Autodesk Inventor part; units mm, degrees
ref_plane "Arbeitsebene1" through (0, -13, 39.6) normal (0, 1, 0) x (-1, 0, 0)
ref_plane "YZ Plane" through (0, 0, 0) normal (1, 0, 0) x (0, 1, 0)
ref_plane "XY Plane" through (0, 0, 0) normal (0, 0, 1) x (1, 0, 0)
sketch "Skizze1" plane through (0, 0, 0) normal (0, 0, 1) x (1, 0, 0)
  circle A0 centre (0, 0) radius 15
  dimension "d0" = 30
extrude "Extrusion1" add sketch "Skizze1" along normal blind 39.6
sketch "Skizze2" plane through (0, 0, 39.6) normal (0, 0, 1) x (1, 0, 0)
  circle A0 centre (0, 0) radius 13
  dimension "d3" = 26
extrude "Extrusion2" add sketch "Skizze2" along normal blind 23
sketch "Skizze5" plane through (0, 0, 62.6) normal (0, 0, 1) x (1, 0, 0)
  circle A0 centre (0, 0) radius 9.2
  dimension "d6" = 18.4
extrude "Extrusion3" cut sketch "Skizze5" against normal through all
sketch "Skizze6" plane through (0, 0, 0) normal (0, 0, -1) x (-1, 0, 0)
  circle A0 centre (0, 0) radius 13.9
  dimension "d9" = 27.8
extrude "Extrusion4" cut sketch "Skizze6" against normal blind 20
ref_plane "Arbeitsebene1" through (0, -13, 39.6) normal (0, 1, 0) x (-1, 0, 0)
sketch "Skizze7" plane through (0, -13, 39.6) normal (0, 1, 0) x (-1, 0, 0)
  line L0 (13, 23) -> (-13, 23)
  line L1 (-9.2, 23) -> (9.2, 23) construction
  line L2 (0, 23) -> (0, 14) construction
  point P0 (0, -39.6)
  dimension "d12" = 9
hole "Bohrung1" at (0, -13, 53.6) direction (0, 1, 0) diameter 2.013 end up to surface
properties part number "tubus lense (423606-8031)"
Verification items for the finished model (mm, model axes). A direction names the side the tool comes from. Round coordinates to 2 decimals unless told otherwise and drop trailing zeros. Order: outer loops, then holes, each group sorted by start corner. A loop starts at its lowest first (then second) coordinate and runs counter-clockwise, first axis right, second up. Notation, with made-up numbers: (82.25, 80.25) -> (98.25, 80.25) arc R20 cw to (98.25, 108.25) -> close; hole circle Ø10 at (14, 31). An arc over 180 degrees is marked (long way). Put each result on its own line as item: value. Start each with the question number.
(1) Draft check along Y on faces 1 (the face through (-14.985, -0.66, 19.523)), 2 (the face through (3, 9, 62.6)), 3 (the face through (-7.3, -5.6, 41.6)). Enter one of: +Y half, -Y half, draft (parallel to the pull), parting line (faces both ways), or undercut.
(2) Section check B-B (y = 0). Enter the section's corners in (x, z).
(3) Depth check by flat-ended pin: pin 1 Ø3 at (y, z) = (2, 41.5) entering from -X; pin 2 Ø2.5 at (x, z) = (0, 53.6) entering from +Y; pin 3 Ø5 at (x, y) = (2, -4) entering from -Z; pin 4 Ø12 at (x, z) = (5, 25) entering from -Y. Enter the tip coordinate at first touch or a pass-through.
(4) Tool access check on faces 4 (the face through (-10.316, 7.91, 50.939)), 5 (the face through (10, -10, 0)), 6 (the face through (-0.3, -11.05, 52.64)), 7 (the face through (-9, -3, 20)). Record the directions out of +Z, -Z, +X, -X, +Y, -Y that give a thin tool (end or side, any length) a straight path to the whole face; none if there is none.
(5) Section check D-D (z = 50). Enter the section's corners in (x, y).
(6) Section check A-A (x = 0). Enter the section's corners in (y, z), then the cut area to 3 significant figures.
(7) Section check C-C (x = -6.25). Enter the section's corners in (y, z), then the cut area to 3 significant figures.
(8) Material ranges on line 1 along Y through (x, z) = (0.5, 56); line 2 along X through (y, z) = (5.25, 51.5); line 3 along Y through (x, z) = (4.25, 14.5), recorded low to high.
Completed:
1. face 1: parting line
1. face 2: draft
1. face 3: undercut
2. outline: (-15, 0) -> (-13.9, 0) -> (-13.9, 20) -> (-9.2, 20) -> (-9.2, 62.6) -> (-13, 62.6) -> (-13, 39.6) -> (-15, 39.6) -> close; (9.2, 20) -> (13.9, 20) -> (13.9, 0) -> (15, 0) -> (15, 39.6) -> (13, 39.6) -> (13, 62.6) -> (9.2, 62.6) -> close
3. pin 1: stops at x = -12.99
3. pin 2: stops at y = 13
3. pin 3: passes through
3. pin 4: stops at y = -15
4. face 4: +Z
4. face 5: -Z, +X, -X, +Y, -Y
4. face 6: -Y
4. face 7: -Z
5. outline: circle Ø26 at (0, 0); hole circle Ø18.4 at (0, 0)
6. outline: (-15, 0) -> (-13.9, 0) -> (-13.9, 20) -> (-9.2, 20) -> (-9.2, 52.59) -> (-13, 52.59) -> (-13, 39.6) -> (-15, 39.6) -> close; (-13, 54.61) -> (-9.2, 54.61) -> (-9.2, 62.6) -> (-13, 62.6) -> close; (9.2, 20) -> (13.9, 20) -> (13.9, 0) -> (15, 0) -> (15, 39.6) -> (13, 39.6) -> (13, 62.6) -> (9.2, 62.6) -> close
6. area: 439 mm2
7. outline: (-13.64, 0) -> (-12.42, 0) -> (-12.42, 20) -> (-6.75, 20) -> (-6.75, 62.6) -> (-11.4, 62.6) -> (-11.4, 39.6) -> (-13.64, 39.6) -> close; (6.75, 20) -> (12.42, 20) -> (12.42, 0) -> (13.64, 0) -> (13.64, 39.6) -> (11.4, 39.6) -> (11.4, 62.6) -> (6.75, 62.6) -> close
7. area: 532 mm2
8. line 1: y = -12.99 to -9.19, 9.19 to 12.99
8. line 2: x = -11.89 to -7.55, 7.55 to 11.89
8. line 3: y = -14.39 to -13.23, 13.23 to 14.39
